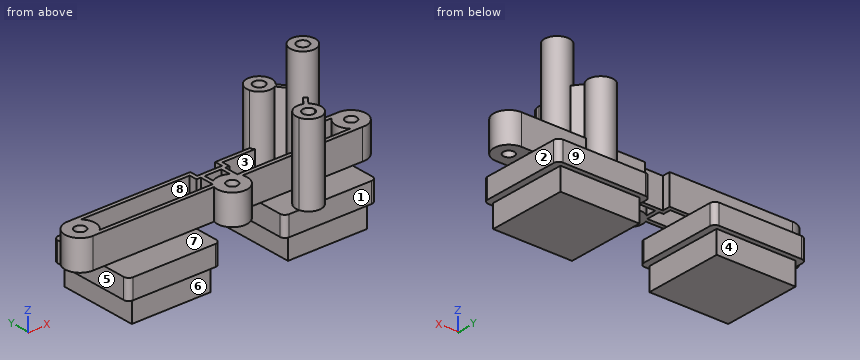
from build123d import *

# Parameters (mm, degrees)
ESQUISSE1_R        = 3
ESQUISSE1_R_2      = 1.1
EXTRUSION1_DEPTH   = 6
EXTRUSION1_2_DEPTH = 6
EXTRUSION1_3_DEPTH = 6
EXTRUSION2_DEPTH   = 6
ESQUISSE3_W        = 15.8
ESQUISSE3_H        = 15.8
EXTRUSION3_DEPTH   = 8.5
EXTRUSION4_DEPTH   = 4
ESQUISSE5_R        = 2.5
ESQUISSE5_R_2      = 1.15
EXTRUSION5_DEPTH   = 24
ESQUISSE6_R        = 2.5
ESQUISSE6_R_2      = 1.15
EXTRUSION6_DEPTH   = 16
EXTRUSION7_DEPTH   = 16


with BuildPart() as part:
    # Esquisse1 → Extrusion1 (new body)
    with BuildSketch(Plane.XY):
        with Locations((-27.15, 42.398738828)):
            Circle(ESQUISSE1_R)
        with Locations((-27.15, 42.398738828)):
            Circle(ESQUISSE1_R_2, mode=Mode.SUBTRACT)
    extrude(amount=EXTRUSION1_DEPTH)



with BuildPart() as body_2:
    # Esquisse1 → Extrusion1 2 (new body)
    with BuildSketch(Plane.XY):
        with Locations((0, 38.498738828)):
            Circle(ESQUISSE1_R)
        with Locations((0, 38.498738828)):
            Circle(ESQUISSE1_R_2, mode=Mode.SUBTRACT)
    extrude(amount=EXTRUSION1_2_DEPTH)


with BuildPart() as body_3:
    # Esquisse1 → Extrusion1 3 (new body)
    with BuildSketch(Plane.XY):
        with Locations((27.15, 42.398738828)):
            Circle(ESQUISSE1_R)
        with Locations((27.15, 42.398738828)):
            Circle(ESQUISSE1_R_2, mode=Mode.SUBTRACT)
    extrude(amount=EXTRUSION1_3_DEPTH)


with BuildPart() as part_1:
    add(part.part)

    add(body_2.part)  # Extrusion2 merges body 2

    add(body_3.part)  # Extrusion2 merges body 3
    # Esquisse2 → Extrusion2 (add)
    with BuildSketch(Plane.XY.offset(6)):
        Polygon((-27.15, 45.398738828), (-2.513675589, 45.398738828), (-2.513675589, 44.598738828), (-2.513675589, 43.7970137), (2.463807407, 43.7970137), (2.463807407, 44.724328248), (2.463807407, 45.398738828), (27.161568979, 45.398738828), (27.161568979, 44.598738828), (3.263807407, 44.598738828), (3.263807407, 42.9970137), (2.463807407, 42.9970137), (2.463807407, 40.21036176), (27.413822862, 40.21036176), (27.413822862, 39.41036176), (2.20772744, 39.41036176), (1.663807407, 39.41036176), (1.663807407, 42.9970137), (-1.671841419, 42.9970137), (-1.671841419, 39.398738828), (-2.471841419, 39.398738828), (-27.15, 39.398738828), (-27.15, 40.198738828), (-2.471841419, 40.198738828), (-2.471841419, 42.9970137), (-3.313675589, 42.9970137), (-3.313675589, 44.598738828), (-27.15, 44.598738828), align=None)
    extrude(amount=-EXTRUSION2_DEPTH)

    # Esquisse3 → Extrusion3 (add)
    with BuildSketch(Plane(origin=(0, 0, 0), x_dir=(-1, 0, 0), z_dir=(0, 0, -1))):
        with Locations((15.65, 42.398738828)):
            Rectangle(ESQUISSE3_W, ESQUISSE3_H)
        with Locations((-15.65, 42.398738828)):
            Rectangle(ESQUISSE3_W, ESQUISSE3_H)
    extrude(amount=EXTRUSION3_DEPTH)

    # Esquisse4 → Extrusion4 (add)
    with BuildSketch(Plane(origin=(0, 0, 0), x_dir=(-1, 0, 0), z_dir=(0, 0, -1))):
        with BuildLine():
            Line((7.4, 33.798738828), (23.9, 33.798738828))
            ThreePointArc((23.9, 33.798738828), (24.607106781, 34.091632046), (24.9, 34.798738828))
            Line((24.9, 34.798738828), (24.9, 50.298738828))
            ThreePointArc((24.9, 50.298738828), (24.607106781, 51.005845609), (23.9, 51.298738828))
            Line((23.9, 51.298738828), (7.4, 51.298738828))
            ThreePointArc((7.4, 51.298738828), (6.692893219, 51.005845609), (6.4, 50.298738828))
            Line((6.4, 50.298738828), (6.4, 34.798738828))
            ThreePointArc((6.4, 34.798738828), (6.692893219, 34.091632046), (7.4, 33.798738828))
        make_face()
        with BuildLine():
            Line((-6.4, 34.798738828), (-6.4, 50.298738828))
            ThreePointArc((-6.4, 50.298738828), (-6.692893219, 51.005845609), (-7.4, 51.298738828))
            Line((-7.4, 51.298738828), (-23.9, 51.298738828))
            ThreePointArc((-23.9, 51.298738828), (-24.607106781, 51.005845609), (-24.9, 50.298738828))
            Line((-24.9, 50.298738828), (-24.9, 34.798738828))
            ThreePointArc((-24.9, 34.798738828), (-24.607106781, 34.091632046), (-23.9, 33.798738828))
            Line((-23.9, 33.798738828), (-7.4, 33.798738828))
            ThreePointArc((-7.4, 33.798738828), (-6.692893219, 34.091632046), (-6.4, 34.798738828))
        make_face()
    extrude(amount=EXTRUSION4_DEPTH)

    # Esquisse5 → Extrusion5 (add)
    with BuildSketch(Plane.XY):
        with Locations(Location((15.605002706, 40.204414181, 0), (0, 0, 179.863691409))):
            Circle(ESQUISSE5_R)
        with Locations(Location((15.605002706, 40.204414181, 0), (0, 0, 179.703675934))):
            Circle(ESQUISSE5_R_2, mode=Mode.SUBTRACT)
    extrude(amount=EXTRUSION5_DEPTH)

    # Esquisse6 → Extrusion6 (add)
    # profile 1 of 5: a face of its own
    with BuildSketch(Plane.XY):
        with BuildLine():
            ThreePointArc((10.827425412, 33.798738828), (11.490132803, 35.510468856), (12.955002706, 34.404414181))
            ThreePointArc((12.955002706, 34.404414181), (12.911057381, 34.089544278), (12.78258, 33.798738828))
            Line((12.78258, 33.798738828), (14.230524787, 33.798738828))
            ThreePointArc((14.230524787, 33.798738828), (14.286313368, 34.099295518), (14.305002706, 34.404414181))
            ThreePointArc((14.305002706, 34.404414181), (11.499884043, 36.885724843), (9.379480625, 33.798738828))
            Line((9.379480625, 33.798738828), (10.827425412, 33.798738828))
        make_face()
    # profile 2 of 5: a face of its own
    with BuildSketch(Plane.XY):
        with BuildLine():
            ThreePointArc((12.78258, 33.798738828), (11.805002706, 33.254414181), (10.827425412, 33.798738828))
            Line((10.827425412, 33.798738828), (9.379480625, 33.798738828))
            ThreePointArc((9.379480625, 33.798738828), (11.805002706, 31.904414181), (14.230524787, 33.798738828))
            Line((14.230524787, 33.798738828), (12.78258, 33.798738828))
        make_face()
    # profile 3 of 5: a face of its own
    with BuildSketch(Plane.XY):
        with BuildLine():
            ThreePointArc((10.827425412, 33.798738828), (11.490132803, 35.510468856), (12.955002706, 34.404414181))
            ThreePointArc((12.955002706, 34.404414181), (12.911057381, 34.089544278), (12.78258, 33.798738828))
            Line((12.78258, 33.798738828), (14.230524787, 33.798738828))
            ThreePointArc((14.230524787, 33.798738828), (14.286313368, 34.099295518), (14.305002706, 34.404414181))
            ThreePointArc((14.305002706, 34.404414181), (11.499884043, 36.885724843), (9.379480625, 33.798738828))
            Line((9.379480625, 33.798738828), (10.827425412, 33.798738828))
        make_face()
    # profile 4 of 5: a face of its own
    with BuildSketch(Plane.XY):
        with BuildLine():
            ThreePointArc((12.78258, 33.798738828), (11.805002706, 33.254414181), (10.827425412, 33.798738828))
            Line((10.827425412, 33.798738828), (9.379480625, 33.798738828))
            ThreePointArc((9.379480625, 33.798738828), (11.805002706, 31.904414181), (14.230524787, 33.798738828))
            Line((14.230524787, 33.798738828), (12.78258, 33.798738828))
        make_face()
    # profile 5 of 5: a face of its own
    with BuildSketch(Plane.XY):
        with Locations(Location((11.805002706, 46.004414181, 0), (0, 0, 194.020564777))):
            Circle(ESQUISSE6_R)
        with Locations(Location((11.805002706, 46.004414181, 0), (0, 0, 211.781019499))):
            Circle(ESQUISSE6_R_2, mode=Mode.SUBTRACT)
    extrude(amount=EXTRUSION6_DEPTH)

    # Esquisse7 → Extrusion7 (add)
    with BuildSketch(Plane.XY.offset(16)):
        Polygon((12.558485139, 36.446515131), (14.292905081, 38.694837279), (14.882025317, 38.240373098), (12.955002706, 35.742380824), align=None)
        Polygon((13.393576222, 44.668950414), (15.320709492, 42.099439388), (14.71430489, 41.644635937), (12.955002706, 43.990372182), align=None)
    extrude(amount=-EXTRUSION7_DEPTH)


solid = part_1.part
Design review of the part built by this model. Coordinates are the model's own, in mm. Face numbers are marked on the shaded views. A direction names the side the tool comes from. Round coordinates to 2 decimals unless told otherwise and drop trailing zeros. Write each loop counter-clockwise with the first axis right and the second up, starting at its lowest first coordinate (ties: lowest second). Pieces come first, ordered by that corner, then holes. Notation, with made-up numbers: (-23, -30.5) -> (21, -30.5) arc R11 ccw to (21, -16.5) -> close; hole circle Ø6 at (6, 1.25). An arc over 180 degrees is marked (long way). One line per item, written item: value. Start each with the question number.
Q1. The part is to be moulded in two halves that separate along Y. For the marked faces 6, 7, 8 and 9, say which applies: pulls with the +Y half, pulls with the -Y half, needs draft (parallel to the pull), parting line crosses it, or undercut.
Q2. Add section D-D (x = -11). Give the boundary of the cut face in (y, z).
Q3. Add section C-C (z = 15). State how many separate pieces and enclosed holes the cut face has, then the cut area to 3 significant figures.
Q4. Add section A-A (z = -1.5). Give the boundary of the cut face in (x, y), then the cut area to 3 significant figures.
Q5. Tool access review of the marked faces 1, 2, 3, 4 and 5: name each direction out of +Z, -Z, +X, -X, +Y, -Y from which nothing blocks a thin tool from reaching the whole face with its end or side.
Q6. Insertion check: P1, Ø1.8, axis at x = 19, y = 42.5, coming from the +Z side; P2, Ø1.8, axis at x = -13, z = 2.5, coming from the +Y side; P3, Ø3, axis at x = 12.5, z = -2.5, coming from the -Y side. Each pin has a flat end and moves straight along its axis. Give the tip position at first contact, or say it passes through.
Q7. Add section B-B (x = 0). Give the boundary of the cut face in (y, z), then the cut area to 3 significant figures.
Q8. To check wall thickness, follow probe 1 along Y at (x, z) = (0, 4); probe 2 along X at (y, z) = (48.25, -4.5); probe 3 along X at (y, z) = (34.25, 8). State the ranges of each line that lie inside material, in increasing order.
Response:
1. face 6: pulls with the -Y half
1. face 7: needs draft
1. face 8: undercut
1. face 9: pulls with the +Y half
2. outline: (33.8, -4) -> (34.5, -4) -> (34.5, -8.5) -> (50.3, -8.5) -> (50.3, -4) -> (51.3, -4) -> (51.3, 0) -> (45.4, 0) -> (45.4, 6) -> (44.6, 6) -> (44.6, 0) -> (40.2, 0) -> (40.2, 6) -> (39.4, 6) -> (39.4, 0) -> (33.8, 0) -> close
3. separate pieces: 1
3. enclosed holes: 3
3. area: 49.4 mm^2
4. outline: (-24.9, 34.8) arc R1 ccw to (-23.9, 33.8) -> (-7.4, 33.8) arc R1 ccw to (-6.4, 34.8) -> (-6.4, 50.3) arc R1 ccw to (-7.4, 51.3) -> (-23.9, 51.3) arc R1 ccw to (-24.9, 50.3) -> close; (6.4, 34.8) arc R1 ccw to (7.4, 33.8) -> (23.9, 33.8) arc R1 ccw to (24.9, 34.8) -> (24.9, 50.3) arc R1 ccw to (23.9, 51.3) -> (7.4, 51.3) arc R1 ccw to (6.4, 50.3) -> close
4. area: 646 mm^2
5. face 1: -Z, +X, -X, -Y
5. face 2: -Z, +X, +Y, -Y
5. face 3: +Z
5. face 4: -Z, +X, -X, +Y
5. face 5: -Z, -X, +Y, -Y
6. P1: stops at z = 0
6. P2: stops at y = 45.4
6. P3: stops at y = 33.8
7. outline: (35.5, 0) -> (37.4, 0) -> (37.4, 6) -> (35.5, 6) -> close; (39.6, 0) -> (41.5, 0) -> (41.5, 6) -> (39.6, 6) -> close; (43, 0) -> (43.8, 0) -> (43.8, 6) -> (43, 6) -> close
7. area: 27.6 mm^2
8. probe 1: y = 35.5 to 37.4, 39.6 to 41.5, 43 to 43.8
8. probe 2: x = -23.55 to -7.75, 7.75 to 23.55
8. probe 3: x = 9.31 to 10.67, 12.94 to 14.3
